from build123d import *

# Parameters (mm, degrees)
F0_W      = 40
F0_H      = 25
F1_DEPTH  = 2
F2_W      = 14
F2_H      = 25
F3_DEPTH  = 30
F5_D      = 4
F6_W      = 11
F6_H      = 17
F7_DEPTH  = 29
F9_DEPTH  = 3
F11_DEPTH = 5
F13_DEPTH = 5


with BuildPart() as f1:
    # F0 (on Top) → F1 (new body)
    with BuildSketch(Plane.XY):
        Rectangle(F0_W, F0_H)
    extrude(amount=F1_DEPTH)

    # F2 (on face) → F3 (join)
    with BuildSketch(Plane.XY.offset(2)):
        Rectangle(F2_W, F2_H)
    extrude(amount=F3_DEPTH)

    # F5 (through all)
    with Locations(Plane.XY.offset(2)):
        with Locations((13.51337, 0), (-13.51337, 0)):
            Hole(F5_D / 2)

    # F6 (on face) → F7 (cut)
    with BuildSketch(Plane(origin=(0, 0, 0), x_dir=(1, 0, 0), z_dir=(0, 0, -1))):
        Rectangle(F6_W, F6_H)
    extrude(amount=-F7_DEPTH, mode=Mode.SUBTRACT)

    # F8 (on face) → F9 (cut)
    with BuildSketch(Plane.XY.offset(32)):
        Polygon((-3.5, -6.5), (0, -6.5), (3.5, -6.5), (3.5, 0), (-3.5, 0), align=None)
    extrude(amount=-F9_DEPTH, mode=Mode.SUBTRACT)

    # F10 (on face) → F11 (cut)
    with BuildSketch(Plane.XZ.offset(12.5)):
        Polygon((-2.5, 0), (0, 0), (2.5, 0), (2.5, 18), (-2.5, 18), align=None)
    extrude(amount=-F11_DEPTH, mode=Mode.SUBTRACT)

    # F12 (on face) → F13 (cut)
    with BuildSketch(Plane(origin=(0, 12.5, 0), x_dir=(-1, 0, 0), z_dir=(0, 1, 0))):
        Polygon((-4, 0), (0, 0), (4, 0), (4, 26), (0, 26), (-4, 26), align=None)
    extrude(amount=-F13_DEPTH, mode=Mode.SUBTRACT)


solid = f1.part
Part model, mm, in its own coordinate system. A direction names the side the tool comes from. Give positions to 0.01 mm unless a question says otherwise; leave off trailing zeros. Loops run counter-clockwise (first coordinate to the right, second up) from the corner with the lowest first, then second, coordinate; pieces in that order, holes last. Notation, with made-up numbers: (37.25, 17.5) -> (71.25, 17.5) arc R20 cw to (71.25, 23.5) -> close; hole circle Ø3 at (31.25, 15). An arc over 180 degrees is marked (long way). Write each question's results on one line, items separated by ' | '. Start each with the question number.
Q1. Band-saw the part on B-B on x = 3. List the corners of the cut face in (y, z), plus the area to 4 significant figures.
Q2. Pin check, flat tips, straight feed: P1, Ø1.5, axis at x = -11.5, y = 7, coming from the -Z side; P2, Ø3.5, axis at x = 1, z = 9, coming from the +Y side; P3, Ø10.5, axis at x = 12.5, y = 5, coming from the +Z side; P4, Ø1.2, axis at y = 10, z = 16, coming from the -X side. Stop position of each tip, or through.
Q3. Wall check: L1, parallel to X at y = 4.75, z = 7; L2, parallel to X at y = -11, z = 6; L3, parallel to Z at x = 8.5, y = 2.25. Give the ranges that are in metal, low to high.
Q4. Band-saw the part on C-C on y = 1.5. List the corners of the cut face in (x, z).
Q5. Band-saw the part on D-D on z = 29.5. List the corners of the cut face in (x, y), plus the area to 4 significant figures.
Q6. Pull direction X, two halves, no side cores. Call faces 1 (the face through (-14, 3, 2)), 2 (the face through (-7, 0, 17)), 3 (the face through (0, 2, 29)): +X half, -X half, draft (parallel to the pull), parting line (faces both ways), or undercut.
Q7. Band-saw the part on A-A on z = 2.5. List the corners of the cut face in (x, y).
Q8. Which spindle directions (+Z, -Z, +X, -X, +Y, -Y) get a long thin tool onto all of the face, cutting with end or side? Do faces 4 (the face through (4, 11, 13)), 5 (the face through (-2.5, -11, 9)), 6 (the face through (0, 0, 31)), 7 (the face through (13, 3, 2)). Say none if no direction does.
Results are:
1) outline: (-12.5, 0) -> (-8.5, 0) -> (-8.5, 29) -> (-6.5, 29) -> (-6.5, 32) -> (-12.5, 32) -> close; (0, 29) -> (8.5, 29) -> (8.5, 26) -> (12.5, 26) -> (12.5, 32) -> (0, 32) -> close | area: 183.5 mm²
2) P1: stops at z = 0 | P2: stops at y = -8.5 | P3: stops at z = 2 | P4: stops at x = -7
3) L1: x = -7 to -5.5, 5.5 to 7 | L2: x = -7 to -2.5, 2.5 to 7 | L3: z = 0 to 2
4) outline: (-20, 0) -> (-14.84, 0) -> (-14.84, 2) -> (-20, 2) -> close; (-12.19, 0) -> (-5.5, 0) -> (-5.5, 29) -> (5.5, 29) -> (5.5, 0) -> (12.19, 0) -> (12.19, 2) -> (7, 2) -> (7, 32) -> (-7, 32) -> (-7, 2) -> (-12.19, 2) -> close; (14.84, 0) -> (20, 0) -> (20, 2) -> (14.84, 2) -> close
5) outline: (-7, -12.5) -> (7, -12.5) -> (7, 12.5) -> (-7, 12.5) -> close; hole (-3.5, -6.5) -> (3.5, -6.5) -> (3.5, 0) -> (-3.5, 0) -> close | area: 304.5 mm²
6) face 1: draft | face 2: -X half | face 3: undercut
7) outline: (-7, -12.5) -> (-2.5, -12.5) -> (-2.5, -8.5) -> (-5.5, -8.5) -> (-5.5, 8.5) -> (-4, 8.5) -> (-4, 12.5) -> (-7, 12.5) -> close; (2.5, -12.5) -> (7, -12.5) -> (7, 12.5) -> (4, 12.5) -> (4, 8.5) -> (5.5, 8.5) -> (5.5, -8.5) -> (2.5, -8.5) -> close
8) face 4: -Z, +Y | face 5: -Z, +Y, -Y | face 6: +Z, -Z | face 7: +Z, +X, +Y, -Y
